Check sheet for the modelled part. Datum: model origin and axes. Units: mm. Give positions to 0.01 mm unless a question says otherwise; leave off trailing zeros. Order: outer loops, then holes, each group sorted by start corner. A loop starts at its lowest first (then second) coordinate and runs counter-clockwise, first axis right, second up. Notation, with made-up numbers: (82, -15.5) -> (88, -15.5) arc R11 ccw to (88, -3.5) -> close; hole circle Ø3 at (18, 33). An arc over 180 degrees is marked (long way). One line per question, with ' | ' between items.
```python
from build123d import *

# Parameters (mm, degrees)
SKETCH1_R           = 1.5
BOSS_EXTRUDE1_DEPTH = 3.18
SKETCH6_R           = 1.5
SKETCH6_W           = 71.2
SKETCH6_H           = 24
CUT_EXTRUDE2_DEPTH  = 10
SKETCH7_R           = 3.4
CUT_EXTRUDE3_DEPTH  = 10
SKETCH8_R           = 6.1
CUT_EXTRUDE4_DEPTH  = 10
SKETCH9_W           = 1.359875129
SKETCH9_H           = 2.955102212
CUT_EXTRUDE5_DEPTH  = 10


with BuildPart() as part:
    # Sketch1 → Boss-Extrude1 (new body)
    with BuildSketch(Plane.XY):
        Polygon((-78.18, 75), (-12.5, 75), (-12.5, 78.18), (12.5, 78.18), (12.5, 75), (78.18, 75), (78.18, 12.5), (75, 12.5), (75, 1.5), (71, 1.5), (71, 4.5), (68, 4.5), (68, 1.5), (65.18, 1.5), (65.18, -1.5), (68, -1.5), (68, -4.5), (71, -4.5), (71, -1.5), (75, -1.5), (75, -12.5), (78.18, -12.5), (78.18, -75), (12.5, -75), (12.5, -78.18), (-12.5, -78.18), (-12.5, -75), (-78.18, -75), (-78.18, -12.5), (-75, -12.5), (-75, -1.5), (-71, -1.5), (-71, -4.5), (-68, -4.5), (-68, -1.5), (-65.18, -1.5), (-65.18, 1.5), (-68, 1.5), (-68, 4.5), (-71, 4.5), (-71, 1.5), (-75, 1.5), (-75, 12.5), (-78.18, 12.5), align=None)
        with Locations(Location((0, -76.59, 0), (0, 0, 180))):
            Circle(SKETCH1_R, mode=Mode.SUBTRACT)
        with Locations(Location((0, 76.59, 0), (0, 0, 180))):
            Circle(SKETCH1_R, mode=Mode.SUBTRACT)
    extrude(amount=BOSS_EXTRUDE1_DEPTH)

    # Sketch6 → Cut-Extrude2 (cut)
    with BuildSketch(Plane.XY.offset(3.18)):
        with Locations((-36.094459363, 18.581758052)):
            Circle(SKETCH6_R)
        with Locations((-36.094459363, -12.418241948)):
            Circle(SKETCH6_R)
        with Locations((38.905540637, -12.418241948)):
            Circle(SKETCH6_R)
        with Locations((38.905540637, 18.581758052)):
            Circle(SKETCH6_R)
        with Locations((1.505540637, 3.581758052)):
            Rectangle(SKETCH6_W, SKETCH6_H)
    extrude(amount=-CUT_EXTRUDE2_DEPTH, mode=Mode.SUBTRACT)

    # Sketch7 → Cut-Extrude3 (cut)
    with BuildSketch(Plane.XY.offset(3.18)):
        with Locations((0, -23.418241948)):
            Circle(SKETCH7_R)
    extrude(amount=-CUT_EXTRUDE3_DEPTH, mode=Mode.SUBTRACT)

    # Sketch8 → Cut-Extrude4 (cut)
    with BuildSketch(Plane.XY.offset(3.18)):
        with Locations((0, 35.581758052)):
            Circle(SKETCH8_R)
    extrude(amount=-CUT_EXTRUDE4_DEPTH, mode=Mode.SUBTRACT)

    # Sketch9 → Cut-Extrude5 (cut)
    with BuildSketch(Plane.XY.offset(3.18)):
        with Locations((-7.96280577, -23.394151807)):
            Rectangle(SKETCH9_W, SKETCH9_H)
    extrude(amount=-CUT_EXTRUDE5_DEPTH, mode=Mode.SUBTRACT)


solid = part.part
```
Q1. Section check A-A (x = 9). Enter the section's corners in (y, z), and give its area (3 significant figures).
Result sheet:
outline: (-78.18, 0) -> (-8.42, 0) -> (-8.42, 3.18) -> (-78.18, 3.18) -> close; (15.58, 0) -> (78.18, 0) -> (78.18, 3.18) -> (15.58, 3.18) -> close | area: 421 mm2
Q2. Section check B-B (x = -50.5). Enter the section's corners in (y, z), and give its area (3 significant figures).
Result sheet:
outline: (-75, 0) -> (75, 0) -> (75, 3.18) -> (-75, 3.18) -> close | area: 477 mm2
Q3. Thickness scan on line 1 (X direction, y = -23, z = 3); line 2 (Y direction, x = -9, z = 2.95); line 3 (Y direction, x = 19, z = 1.55). Record the ranges inside material, lowest first.
Result sheet:
line 1: x = -78.18 to -8.64, -7.28 to -3.37, 3.37 to 78.18 | line 2: y = -78.18 to -8.42, 15.58 to 78.18 | line 3: y = -75 to -8.42, 15.58 to 75
Q4. Mould release check, pull along Y, two halves, no side actions. Record for faces 1 (the face through (-1.322, 29.627, 1.612)), 2 (the face through (1, -16, 0)): pulls with the +Y half, pulls with the -Y half, needs draft (parallel to the pull), parting line crosses it, or undercut.
Result sheet:
face 1: undercut | face 2: needs draft
Q5. Section check C-C (z = 2.45). Count the separate pieces of the cut face and the enclosed holes in it, and give its area (3 significant figures).
Result sheet:
separate pieces: 1 | enclosed holes: 10 | area: 21,500 mm2
Q6. Depth check by flat-ended pin: pin 1 Ø1 at (y, z) = (2, 1) entering from -X; pin 2 Ø1 at (x, z) = (-56.5, 2) entering from -Y; pin 3 Ø1.6 at (y, z) = (-76, 2.5) entering from +X. Enter the tip coordinate at first touch or a pass-through.
Result sheet:
pin 1: stops at x = -75 | pin 2: stops at y = -75 | pin 3: stops at x = 12.5
